Model file for the job. Use its own axes, mm. A direction names the side the tool comes from. Coordinates: 2 decimals unless noted, no trailing zeros. Order: outer loops, then holes, each group sorted by start corner. A loop starts at its lowest first (then second) coordinate and runs counter-clockwise, first axis right, second up. Notation, with made-up numbers: M -15,84 L 3,84 A22 ccw 3,118 Z; hole C 16.5,-38.75 d3. An arc over 180 degrees is marked long. Return JSON: item names as keys, results as strings.
```python
from build123d import *

# Parameters (mm, degrees)
BOSS_EXTRUDE1_DEPTH = 12.7
SKETCH2_W           = 6.35
SKETCH2_H           = 6.35
BOSS_EXTRUDE2_DEPTH = 48.26
BOSS_EXTRUDE3_DEPTH = 12.7
SKETCH4_R           = 5.207
BOSS_EXTRUDE4_DEPTH = 6.35
FILLET1_R           = 2.54


with BuildPart() as part:
    # Sketch1 → Boss-Extrude1 (new body)
    with BuildSketch(Plane.XY):
        Polygon((0, 0), (-12.3952, 0), (-12.3952, 11.43), (-42.6212, 43.18), (-42.6212, 49.53), (-36.2712, 49.53), (0, 11.43), align=None)
    extrude(amount=BOSS_EXTRUDE1_DEPTH)

    # Sketch2 → Boss-Extrude2 (add)
    with BuildSketch(Plane.XY.offset(12.7)):
        with Locations((-39.4462, 46.355)):
            Rectangle(SKETCH2_W, SKETCH2_H)
    extrude(amount=BOSS_EXTRUDE2_DEPTH)

    # Sketch3 → Boss-Extrude3 (add)
    with BuildSketch(Plane.XY.offset(60.96)):
        Polygon((-42.6212, 43.18), (-12.3952, 11.43), (-12.3952, 0), (0, 0), (0, 11.43), (-36.2712, 49.53), (-42.6212, 49.53), align=None)
    extrude(amount=BOSS_EXTRUDE3_DEPTH)

    # Sketch4 → Boss-Extrude4 (add)
    with BuildSketch(Plane(origin=(0, 49.53, 0), x_dir=(1, 0, 0), z_dir=(0, 1, 0))):
        with BuildLine():
            Line((-42.6212, -27.94), (-76.9112, -27.94))
            ThreePointArc((-76.9112, -27.94), (-85.8012, -36.83), (-76.9112, -45.72))
            Line((-76.9112, -45.72), (-42.6212, -45.72))
            Line((-42.6212, -45.72), (-42.6212, -27.94))
        make_face()
        with Locations((-76.9112, -36.83)):
            Circle(SKETCH4_R, mode=Mode.SUBTRACT)
    extrude(amount=-BOSS_EXTRUDE4_DEPTH)

    # Fillet1
    fillet1_edges = [part.edges().sort_by_distance(p)[0] for p in [
        (-39.4462, 43.18, 12.7),
        (-36.2712, 46.355, 12.7),
        (-39.4462, 43.18, 60.96),
        (-36.2712, 46.355, 60.96),
        (-42.6212, 46.355, 45.72),
        (-42.6212, 46.355, 27.94),
    ]]
    fillet(fillet1_edges, radius=FILLET1_R)


solid = part.part
```
Item 1: Wall check: line 1 (X direction, y = 47.25, z = 36.83); line 2 (Z direction, x = -8, y = 4); line 3 (Y direction, x = -73.5, z = 42). Give the ranges that are in metal, low to high.
Check result:
{"line 1": "x = -85.8 to -82.12, -71.7 to -36.27", "line 2": "z = 0 to 12.7, 60.96 to 73.66", "line 3": "y = 43.18 to 49.53"}
Item 2: Drop flat-ended pins along their axis: pin 1 Ø1.9 at (x, y) = (-68, 47.5) entering from +Z; pin 2 Ø3 at (x, y) = (-69, 47.5) entering from -Z; pin 3 Ø6 at (y, z) = (35, 9.5) entering from -X. Give the stop position or say it passes through.
Check result:
{"pin 1": "stops at z = 45.72", "pin 2": "stops at z = 27.94", "pin 3": "stops at x = -37.69"}
Item 3: Pull direction Z, two halves, no side cores. Call faces 6 (the flat face through (-36.271, 46, 37)), 7 (the flat face through (0, 6, 67)), 8 (the cylindrical face through (-43.35, 46.31, 27.18)): +Z half, -Z half, draft (parallel to the pull), parting line (faces both ways), or undercut.
Check result:
{"face 6": "undercut", "face 7": "draft", "face 8": "-Z half"}
Item 4: 3-axis set-ups, long thin cutter, end or side, ignore diameter. For faces 1 (the cylindrical face through (-35.547, 45.147, 13.464)), 2 (the flat face through (-6, 0, 67)), 3 (the flat face through (-42.621, 46, 13)), 4 (the flat face through (-12.395, 6, 67)), 5 (the cylindrical face through (-38.114, 42.416, 60.236)): which of +Z, -Z, +X, -X, +Y, -Y reach the whole face in a straight line?
Check result:
{"face 1": "+X, +Y, -Y", "face 2": "+Z, -Z, +X, -X, -Y", "face 3": "-Z, -X, +Y, -Y", "face 4": "+Z, -Z, -X, -Y", "face 5": "+X, -X, -Y"}
Item 5: Saw through at B-B (y = 30). Write the cut outline in (x, z).
Check result:
{"outline": "M -30.07,0 L -17.68,0 L -17.68,12.7 L -30.07,12.7 Z; M -30.07,60.96 L -17.68,60.96 L -17.68,73.66 L -30.07,73.66 Z"}
Item 6: Saw through at C-C (z = 63.5). Write the cut outline in (x, y), and give its area (3 significant figures).
Check result:
{"outline": "M -42.62,43.18 L -12.4,11.43 L -12.4,0 L 0,0 L 0,11.43 L -36.27,49.53 L -42.62,49.53 Z", "area": "595 mm2"}
Item 7: Saw through at A-A (z = 36.83). Write the cut outline in (x, y).
Check result:
{"outline": "M -85.8,43.18 L -82.12,43.18 L -82.12,49.53 L -85.8,49.53 Z; M -71.7,43.18 L -36.27,43.18 L -36.27,49.53 L -71.7,49.53 Z"}
Item 8: Saw through at D-D (x = -51.5). Write the cut outline in (y, z).
Check result:
{"outline": "M 43.18,27.94 L 49.53,27.94 L 49.53,45.72 L 43.18,45.72 Z"}
